Part model, mm, in its own coordinate system. A direction names the side the tool comes from. Round coordinates to 2 decimals unless told otherwise and drop trailing zeros. Order: outer loops, then holes, each group sorted by start corner. A loop starts at its lowest first (then second) coordinate and runs counter-clockwise, first axis right, second up. Notation, with made-up numbers: (14, -33.75) - (54, -33.75) arc R22 cw to (54, -23.75) - close; hole circle Ø6 at (-28, 72.25). An arc over 180 degrees is marked (long way). Answer as a JSON object with one key per item and string values.
Autodesk Inventor part; units mm, degrees
ref_plane "YZ Plane" through (0, 0, 0) normal (1, 0, 0) x (0, 1, 0)
ref_plane "XZ Plane" through (0, 0, 0) normal (0, 1, 0) x (-1, 0, 0)
ref_plane "XY Plane" through (0, 0, 0) normal (0, 0, 1) x (1, 0, 0)
sketch "Sketch3" plane through (0, 0, 0) normal (0, 1, 0) x (-1, 0, 0)
  line L0 (0, 0) -> (25, 0)
  line L1 (25, 0) -> (25, -33)
  line L2 (25, -33) -> (0, -33)
  line L3 (0, -33) -> (0, 0)
  dimension "d6" = 25
  dimension "d7" = 33
extrude "Extrusion2" add sketch "Sketch3" along normal blind 2
sketch "Sketch4" plane through (0, 2, 0) normal (0, 1, 0) x (1, 0, 0)
  circle A0 centre (-4, 4) radius 1.5
  line L0 (0, 0) -> (0, 33)
  line L1 (-25, 0) -> (0, 0)
  circle A1 centre (-4, 29) radius 1.5
  line L2 (0, 33) -> (-25, 33)
  circle A2 centre (-20, 4) radius 1.5
  line L3 (-25, 33) -> (-25, 0)
  circle A3 centre (-20, 29) radius 1.5
  dimension "d16" = 3
  dimension "d17" = 4
  dimension "d18" = 4
  dimension "d19" = 3
  dimension "d20" = 4
  dimension "d21" = 4
  dimension "d22" = 3
  dimension "d23" = 16
  dimension "d24" = 4
  dimension "d25" = 5
  dimension "d26" = 3
  dimension "d27" = 4
  dimension "d28" = 16
  dimension "d29" = 25
extrude "Extrusion3" cut sketch "Sketch4" against normal blind 2 contours A0 | A1 | A2 | A3
sketch "Sketch5" plane through (0, 2, 0) normal (0, 1, 0) x (1, 0, 0)
  line L0 (-16, 11) -> (-9, 11)
  line L1 (-9, 11) -> (-9, 14)
  line L2 (-9, 14) -> (-16, 14)
  line L3 (-16, 14) -> (-16, 11)
  line L4 (-25, 33) -> (-25, 0)
  line L5 (0, 0) -> (0, 33)
  line L6 (-25, 0) -> (0, 0)
  line L7 (0, 33) -> (-25, 33)
  circle A0 centre (-4, 29) radius 1.5
  circle A1 centre (-20, 29) radius 1.5
  circle A2 centre (-4, 4) radius 1.5
  circle A3 centre (-20, 4) radius 1.5
  line L8 (0, 33) -> (-25, 33)
  line L9 (-25, 33) -> (-25, 0)
  line L10 (-25, 0) -> (0, 0)
  line L11 (0, 0) -> (0, 33)
  line L12 (-16, 19) -> (-9, 19)
  line L13 (-9, 19) -> (-9, 22)
  line L14 (-9, 22) -> (-16, 22)
  line L15 (-16, 22) -> (-16, 19)
  dimension "d32" = 7
  dimension "d36" = 11
  dimension "d37" = 3
  dimension "d39" = 7
  dimension "d40" = 3
  dimension "d41" = 11
  dimension "d42" = 9
  dimension "d43" = 9
extrude "Extrusion4" add sketch "Sketch5" along normal blind 10 contours L3 L2 L1 L0 | L15 L14 L13 L12
sketch "Sketch6" plane through (-16, 2, -11) normal (0, 0, 1) x (1, 0, 0)
  circle A0 centre (3.5, 6.2876) radius 1.5
  line L0 (0, 0) -> (0, 10)
  line L1 (7, 0) -> (7, 10)
  point P0 (16, -2)
  dimension "d46" = 3
  dimension "d47" = 3.5
  dimension "d51" = 3.5
extrude "Extrusion5" cut sketch "Sketch6" against normal blind 13.5
fillet "Fillet1" radius 3 4 edges at (-9, 12, -20.5) (-9, 12, -12.5) (-16, 12, -12.5) (-16, 12, -20.5)
properties part number "CamBracket"
Item 1: Drop flat-ended pins along their axis: P1, Ø1, axis at x = -18, z = -22, coming from the -Y side; P2, Ø4, axis at x = -13.5, y = 10.5, coming from the +Z side; P3, Ø4, axis at x = -20, z = -4, coming from the +Y side; P4, Ø1.5, axis at y = 5.5, z = -12.5, coming from the +X side. Give the stop position or say it passes through.
Taken from the geometry:
{"P1": "y = 0", "P2": "z = -11", "P3": "y = 2", "P4": "x = -9"}
Item 2: Cut at C-C (z = -29). Write the cut outline in (x, y).
Taken from the geometry:
{"outline": "(-25, 0) - (-21.5, 0) - (-21.5, 2) - (-25, 2) - close; (-18.5, 0) - (-5.5, 0) - (-5.5, 2) - (-18.5, 2) - close; (-2.5, 0) - (0, 0) - (0, 2) - (-2.5, 2) - close"}
Item 3: Tool access for faces 4 (the flat face through (-13, 6, -19)), 5 (the flat face through (-16, 5, -21)), 6 (the flat face through (-9, 5, -20)): list every direction of +Z, -Z, +X, -X, +Y, -Y with a clear straight run to the whole face (end or side of a thin tool).
Taken from the geometry:
{"face 4": "+X, -X, +Y", "face 5": "+Z, -Z, -X, +Y", "face 6": "+Z, -Z, +X, +Y"}
Item 4: Cut at B-B (x = -12.5). Write the cut outline in (y, z), plus the area to 3 significant figures.
Taken from the geometry:
{"outline": "(0, -33) - (2, -33) - (2, -22) - (6.79, -22) - (6.79, -19) - (2, -19) - (2, -14) - (6.79, -14) - (6.79, -11) - (2, -11) - (2, 0) - (0, 0) - close; (9.79, -22) - (12, -22) - (12, -19) - (9.79, -19) - close; (9.79, -14) - (12, -14) - (12, -11) - (9.79, -11) - close", "area": "108 mm2"}
Item 5: Probe L1, parallel to X at y = 1.5, z = -29; L2, parallel to Z at x = -20, y = 0.55; L3, parallel to Y at x = -12.5, z = -19.75. List the from-to ranges inside material, lowest first. Write a range as from..to.
Taken from the geometry:
{"L1": "-25..-21.5, -18.5..-5.5, -2.5..0", "L2": "-33..-30.5, -27.5..-5.5, -2.5..0", "L3": "0..6.79, 9.79..12"}
Item 6: Cut at A-A (y = 2.75). Write the cut outline in (x, z).
Taken from the geometry:
{"outline": "(-16, -22) - (-9, -22) - (-9, -19) - (-16, -19) - close; (-16, -14) - (-9, -14) - (-9, -11) - (-16, -11) - close"}
Item 7: Cut at D-D (x = -20). Write the cut outline in (y, z).
Taken from the geometry:
{"outline": "(0, -33) - (2, -33) - (2, -30.5) - (0, -30.5) - close; (0, -27.5) - (2, -27.5) - (2, -5.5) - (0, -5.5) - close; (0, -2.5) - (2, -2.5) - (2, 0) - (0, 0) - close"}
Item 8: Two-plate mould, pull along X, no slides. Class faces 1 (the cylindrical face through (-4.195, 1.014, -30.487)), 2 (the flat face through (-9, 5, -12)), 3 (the flat face through (-13, 1, -33)): pulls with the +X half, pulls with the -X half, needs draft (parallel to the pull), parting line crosses it, or undercut.
Taken from the geometry:
{"face 1": "undercut", "face 2": "pulls with the +X half", "face 3": "needs draft"}
